Geometry check sheet. Reference: the model listing, model coordinates, mm. A direction names the side the tool comes from. Round coordinates to 2 decimals unless told otherwise and drop trailing zeros. Write each loop counter-clockwise with the first axis right and the second up, starting at its lowest first coordinate (ties: lowest second). Pieces come first, ordered by that corner, then holes. Notation, with made-up numbers: M 30,60 L 51,60 A9 ccw 51,75 Z; hole C 66,29 d5. An arc over 180 degrees is marked long. Answer as CSV lines item,"result". Start each with the question number.
```python
from build123d import *

# Parameters (mm, degrees)
F1_DEPTH = 49.5
F2_T     = -2
F3_W     = 45.5
F3_H     = 30.895506
F4_DEPTH = 25
F5_R     = 1.5
F6_DEPTH = 25


with BuildPart() as f1:
    # F0 (on Right) → F1 (new body)
    with BuildSketch(Plane.YZ):
        Polygon((14.57045, 3.255325), (-9.091535, 3.255325), (-9.091535, -65.282837), (-6.643743, -65.282837), (14.57045, -30.197826), align=None)
    extrude(amount=F1_DEPTH)

    # F2
    f2_openings = [f1.faces().sort_by_distance(p)[0] for p in [
        (24.75, -9.091535, -31.013756),
    ]]
    offset(amount=F2_T, openings=f2_openings)

    # F3 (on face) → F4 (cut)
    with BuildSketch(Plane.XZ.offset(-12.57045)):
        with Locations((24.75, -14.192428)):
            Rectangle(F3_W, F3_H)
    extrude(amount=-F4_DEPTH, mode=Mode.SUBTRACT)

    # F5 (on face) → F6 (cut)
    with BuildSketch(Plane(origin=(0, 24.040368, -14.536037), x_dir=(-1, 0, 0), z_dir=(0, 0.855732, -0.517419))):
        with Locations((-43.25, -29.302213)):
            Circle(F5_R)
        with Locations((-43.25, -39.002213)):
            Circle(F5_R)
        with Locations((-43.25, -48.702213)):
            Circle(F5_R)
        with Locations((-6.25, -29.302213)):
            Circle(F5_R)
        with Locations((-6.25, -39.002213)):
            Circle(F5_R)
        with Locations((-6.25, -48.702213)):
            Circle(F5_R)
    extrude(amount=-F6_DEPTH, mode=Mode.SUBTRACT)


solid = f1.part
```
1) Section check B-B, the plane x = 33.5. Record the cut outline in (y, z), plus the area to 3 significant figures.
2) Section check A-A, the plane z = -9. Record the cut outline in (x, y), plus the area to 3 significant figures.
3) Scan lines: line 1 (X direction, y = 3, z = -47.5); line 2 (X direction, y = 10.5, z = -20); line 3 (Z direction, x = 22, y = -8). Record each from-to range of solid material in increasing order. Write a range as from..to.
4) Go/stop test with flat-tipped pins: pin 1 (3 mm diameter, centred on x = 40, z = -47, fed in from +Y); pin 2 (1 mm diameter, centred on x = 43.5, z = -53, fed in from -Y); pin 3 (3 mm diameter, centred on x = 14.5, z = -42.5, fed in from -Y). Record where each tip stops, or that it passes through.
5) Section check D-D, the plane z = -35.5. Record the cut outline in (x, y), plus the area to 3 significant figures.
6) Access from +Z, -Z, +X, -X, +Y, -Y to the whole of each face (thin tool, end or side, straight path). Record for faces 1 (the flat face through (24, 3, 3.255)), 2 (the flat face through (24, -8, -63.283)), 3 (the flat face through (24, 14, -29.64)).
7) Mould release check, pull along X, two halves, no side actions. Record for faces 4 (the flat face through (49.5, 0, -23)), 5 (the flat face through (24, -8, -65.283)), 6 (the flat face through (24.432, 2.257, -46.697)), 7 (the flat face through (47.5, 0, -23)): released by +X, released by -X, zero draft, split by the parting line, or undercut.
8) Section check C-C, the plane y = -5.5. Record the cut outline in (x, z), plus the area to 3 significant figures.
Results:
1,outline,"M -9.09,-65.28 L -6.64,-65.28 L 14.57,-30.2 L 14.57,-29.64 L 12.57,-29.64 L -7.77,-63.28 L -9.09,-63.28 Z; M -9.09,1.26 L 14.57,1.26 L 14.57,3.26 L -9.09,3.26 Z"
1,area,"132 mm^2"
2,outline,"M 0,-9.09 L 2,-9.09 L 2,14.57 L 0,14.57 Z; M 47.5,-9.09 L 49.5,-9.09 L 49.5,14.57 L 47.5,14.57 Z"
2,area,"94.6 mm^2"
3,line 1,"x = 0..4.75, 7.75..41.75, 44.75..49.5"
3,line 2,"x = 0..2, 47.5..49.5"
3,line 3,"z = -65.28..-63.28, 1.26..3.26"
4,pin 1,"stops at y = 5.32"
4,pin 2,"stops at y = -1.86"
4,pin 3,"stops at y = 3.89"
5,outline,"M 0,-9.09 L 2,-9.09 L 2,9.03 L 47.5,9.03 L 47.5,-9.09 L 49.5,-9.09 L 49.5,11.36 L 0,11.36 Z"
5,area,"188 mm^2"
6,face 1,"+Z, +X, -X, +Y, -Y"
6,face 2,"-Y"
6,face 3,"+Y, -Y"
7,face 4,"released by +X"
7,face 5,"zero draft"
7,face 6,"undercut"
7,face 7,"undercut"
8,outline,"M 0,-63.39 L 49.5,-63.39 L 49.5,3.26 L 0,3.26 Z; hole M 2,-59.53 L 47.5,-59.53 L 47.5,1.26 L 2,1.26 Z"
8,area,"533 mm^2"
